The model under review builds one solid part; all positions refer to its coordinate system, in mm. Coordinates: 2 decimals unless noted, no trailing zeros. Order: outer loops, then holes, each group sorted by start corner. A loop starts at its lowest first (then second) coordinate and runs counter-clockwise, first axis right, second up. Notation, with made-up numbers: (79.25, -6) -> (86.25, -6) arc R15 cw to (86.25, 2) -> close; hole circle Ø3 at (38, -28). An arc over 180 degrees is marked (long way). Use CSV: the item, a comma, the result in double quotes. Start each with the question number.
Solid Edge part; units mm, degrees
sketch "Sketch1" plane through (0, 0, 0) normal (1, 0, 0) x (0, 1, 0)
  circle A0 centre (0, 0) radius 2
extrude "Protrusion1" add sketch "Sketch1" along normal mid plane 18
chamfer "Chamfer_1" distance 0.5 angle 45 2 edges at (9, -2, 0) (-9, -2, 0)
sketch "Sketch2" plane through (0, 0, 0) normal (0, -1, 0) x (1, 0, 0)
  line L0 (6, 2) -> (6.5, 2)
  line L1 (6.5, 2) -> (6.5, 1.5)
  line L2 (6.5, 1.5) -> (6, 1.5)
  line L3 (6, 1.5) -> (6, 2)
revolve "RevolvedCutout1" cut sketch "Sketch2" angle 360 about axis through (9, 0, 0) along (-1, 0, 0)
mirror "Mirror1" about plane through (0, 0, 0) normal (1, 0, 0) of "RevolvedCutout1"
properties material "PVC"
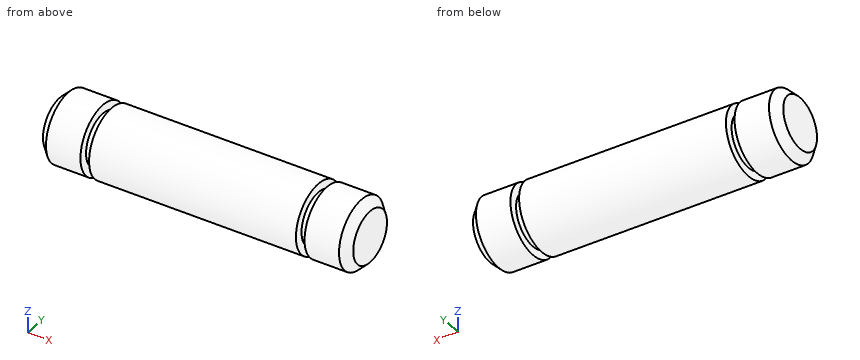
Q1. Add section A-A, the plane z = 0. State the section outline as (x, y) points, then the cut area to 3 significant figures.
Q2. Add section C-C, the plane x = -7.5. State the section outline as (y, z) points.
Q3. To check wall thickness, follow probe 1 along X at (y, z) = (1.4, -0.7); probe 2 along X at (y, z) = (1.4, 1.1); probe 3 along Z at (x, y) = (3.25, 0.1). State the ranges of each line that lie inside material, in increasing order.
Answer block:
1,outline,"(-9, -1.5) -> (-8.5, -2) -> (-6.5, -2) -> (-6.5, -1.5) -> (-6, -1.5) -> (-6, -2) -> (6, -2) -> (6, -1.5) -> (6.5, -1.5) -> (6.5, -2) -> (8.5, -2) -> (9, -1.5) -> (9, 1.5) -> (8.5, 2) -> (6.5, 2) -> (6.5, 1.5) -> (6, 1.5) -> (6, 2) -> (-6, 2) -> (-6, 1.5) -> (-6.5, 1.5) -> (-6.5, 2) -> (-8.5, 2) -> (-9, 1.5) -> close"
1,area,"70.5 mm²"
2,outline,"circle Ø4 at (0, 0)"
3,probe 1,"x = -8.93 to -6.5, -6 to 6, 6.5 to 8.93"
3,probe 2,"x = -8.72 to -6.5, -6 to 6, 6.5 to 8.72"
3,probe 3,"z = -2 to 2"
